Geometry check sheet. Reference: the model listing, model coordinates, mm. A direction names the side the tool comes from. Coordinates: 2 decimals unless noted, no trailing zeros. Write each loop counter-clockwise with the first axis right and the second up, starting at its lowest first coordinate (ties: lowest second). Pieces come first, ordered by that corner, then holes. Notation, with made-up numbers: (-5.5, 9.5) -> (21.5, 9.5) arc R7 ccw to (21.5, 15.5) -> close; hole circle Ø7 at (19, 0). An arc over 180 degrees is marked (long way). Answer in a Markdown table with one row per item. Add a question column.
Q1. Tool access check on faces 1 (the face through (2, 5, 55)), 2 (the face through (-4.032, -6.324, 2.535)), 3 (the face through (6, -16, 57)). Record the directions out of +Z, -Z, +X, -X, +Y, -Y that give a thin tool (end or side, any length) a straight path to the whole face; none if there is none.
Q2. Section check A-A, the plane x = 0. Record the boundary of the cut face in (y, z).
Q3. Thickness scan on line 1 (Y direction, x = 0, z = 56); line 2 (Z direction, x = 7.5, y = 16); line 3 (Y direction, x = -4, z = 40). Record the ranges inside material, lowest first.
Q4. Section check C-C, the plane z = 51. Record the boundary of the cut face in (x, y), and give its area (3 significant figures).
Q5. Gauge pin test, flat ends, axial feed: P1, Ø13, axis at x = 0, y = 0, coming from the -Z side; P2, Ø8, axis at x = 0.5, z = 52.5, coming from the +Y side; P3, Ø6, axis at x = -9.5, z = 33, coming from the +Y side. Record the tip position at first contact, or that the pin passes through.
Q6. Release check for a two-part mould opening along X. For faces 4 (the face through (-2, 5, 5)), 5 (the face through (-6, -16, 3)), 6 (the face through (-15.738, -4.956, 29.622)) record: pulls with the +X half, pulls with the -X half, needs draft (parallel to the pull), parting line crosses it, or undercut.
```python
from build123d import *

# Parameters (mm, degrees)
FILLET_2_R = 1


with BuildPart() as part:
    # 草图1 → 旋转1 (revolve)
    with BuildSketch(Plane(origin=(0, 0, 0), x_dir=(1, 0, 0), z_dir=(0, 1, 0)), mode=Mode.PRIVATE) as revolve_1_sk:
        Polygon((7.5, -55), (7.5, -60), (20, -60), (20, -57), (16.5, -57), (16.5, -3), (20, -3), (20, 0), (7.5, 0), (7.5, -5), (5, -5), (5, -55), align=None)
    revolve(revolve_1_sk.sketch.rotate(Axis((0, 0, 0), (0, 0, 1)), 180), axis=Axis((0, 0, 0), (0, 0, 1)))

    # 圆角2
    fillet_2_edges = [part.edges().sort_by_distance(p)[0] for p in [
        (20, 0, 3),
        (20, 0, 57),
    ]]
    fillet(fillet_2_edges, radius=FILLET_2_R)


solid = part.part
```
Calculated:
| question | item | result |
|---|---|---|
| 1 | face 1 | +Z |
| 1 | face 2 | -Z |
| 1 | face 3 | none |
| 2 | outline | (-20, 0) -> (-7.5, 0) -> (-7.5, 5) -> (-5, 5) -> (-5, 55) -> (-7.5, 55) -> (-7.5, 60) -> (-20, 60) -> (-20, 58) arc R1 ccw to (-19, 57) -> (-16.5, 57) -> (-16.5, 3) -> (-19, 3) arc R1 ccw to (-20, 2) -> close; (5, 5) -> (7.5, 5) -> (7.5, 0) -> (20, 0) -> (20, 2) arc R1 ccw to (19, 3) -> (16.5, 3) -> (16.5, 57) -> (19, 57) arc R1 ccw to (20, 58) -> (20, 60) -> (7.5, 60) -> (7.5, 55) -> (5, 55) -> close |
| 3 | line 1 | y = -16.5 to -7.5, 7.5 to 16.5 |
| 3 | line 2 | z = 0 to 3, 57 to 60 |
| 3 | line 3 | y = -16.01 to -3, 3 to 16.01 |
| 4 | outline | circle Ø33 at (0, 0); hole circle Ø10 at (0, 0) |
| 4 | area | 777 mm² |
| 5 | P1 | stops at z = 5 |
| 5 | P2 | stops at y = 16.5 |
| 5 | P3 | stops at y = 15.17 |
| 6 | face 4 | undercut |
| 6 | face 5 | needs draft |
| 6 | face 6 | parting line crosses it |
